from build123d import *

# Parameters (mm, degrees)
SKETCH_1_R          = 2.75
SKETCH_1_R_2        = 0.75
EXTRUDE_1_DEPTH     = 5.5
SKETCH_2_R          = 0.75
CUT_EXTRUDE_1_DEPTH = 2.75


with BuildPart() as part:
    # 草图1 → 凸台-拉伸1 (new body)
    with BuildSketch(Plane.XY):
        Circle(SKETCH_1_R)
        Circle(SKETCH_1_R_2, mode=Mode.SUBTRACT)
    extrude(amount=EXTRUDE_1_DEPTH)

    # 草图2 → 切除-拉伸1 (cut, symmetric)
    with BuildSketch(Plane(origin=(0, 0, 0), x_dir=(1, 0, 0), z_dir=(0, 1, 0))):
        with Locations((0, -2.75)):
            Circle(SKETCH_2_R)
    extrude(amount=CUT_EXTRUDE_1_DEPTH, both=True, mode=Mode.SUBTRACT)


solid = part.part
Geometry: final body of the model. Coordinates: model frame, mm. Give positions to 0.01 mm unless a question says otherwise; leave off trailing zeros. Write each loop counter-clockwise with the first axis right and the second up, starting at its lowest first coordinate (ties: lowest second). Pieces come first, ordered by that corner, then holes.
(1) Ray query, line 1 (Z direction, x = 0, y = -1.95); line 2 (Y direction, x = 0, z = 4.8); line 3 (X direction, y = -0.45, z = 1.3). Return the intervals inside material, ascending.
(2) Cut plane A-A, the plane x = 0. Return loops of the section in (y, z).
(3) Cut plane C-C, the plane y = 0.15. Return loops of the section in (x, z), then the cut area to 3 significant figures.
(4) Cut plane D-D, the plane z = 1.1. Return loops of the section in (x, y).
(5) Mould query, pull axis X, two halves, no side actions, for faces 1 (the cylindrical face through (1.27, -2.44, 2.71)), 2 (the flat face through (1, -1, 0)), 3 (the cylindrical face through (-0.595, -0.456, 1.05)). Classes: released by +X, released by -X, zero draft, split by the parting line, or undercut.
(6) Cut plane B-B, the plane y = -1.65. Return loops of the section in (x, z).
Values follow:
1. line 1: z = 0 to 2, 3.5 to 5.5
1. line 2: y = -2.75 to -0.75, 0.75 to 2.75
1. line 3: x = -2.71 to -0.6, 0.6 to 2.71
2. outline: (-2.75, 0) - (-0.75, 0) - (-0.75, 2) - (-2.75, 2) - close; (-2.75, 3.5) - (-0.75, 3.5) - (-0.75, 5.5) - (-2.75, 5.5) - close; (0.75, 0) - (2.75, 0) - (2.75, 2) - (0.75, 2) - close; (0.75, 3.5) - (2.75, 3.5) - (2.75, 5.5) - (0.75, 5.5) - close
3. outline: (-2.75, 0) - (-0.73, 0) - (-0.73, 2.6) arc R0.75 cw to (-0.73, 2.9) - (-0.73, 5.5) - (-2.75, 5.5) - close; (0.73, 0) - (2.75, 0) - (2.75, 5.5) - (0.73, 5.5) - (0.73, 2.9) arc R0.75 cw to (0.73, 2.6) - close
3. area: 22.1 mm2
4. outline: circle Ø5.5 at (0, 0); hole circle Ø1.5 at (0, 0)
5. face 1: split by the parting line
5. face 2: zero draft
5. face 3: undercut
6. outline: (-2.2, 0) - (2.2, 0) - (2.2, 5.5) - (-2.2, 5.5) - close; hole circle Ø1.5 at (0, 2.75)
